Read the model definition and answer for the solid it produces. Units are mm, in the model's axes. A direction names the side the tool comes from. Coordinates: 2 decimals unless noted, no trailing zeros. Loops run counter-clockwise (first coordinate to the right, second up) from the corner with the lowest first, then second, coordinate; pieces in that order, holes last. Notation, with made-up numbers: (-5, 35) - (35, 35) arc R27 cw to (35, 62) - close; hole circle Ø8 at (-24, 55). An arc over 180 degrees is marked (long way). One line per item, written item: value. Start each with the question number.
from build123d import *

# Parameters (mm, degrees)
F0_R     = 10.9855
F1_DEPTH = 6.35


with BuildPart() as f1:
    # F0 (on Front) → F1 (new body)
    with BuildSketch(Plane.XZ):
        with BuildLine():
            ThreePointArc((-22.3335889539, 39.0903010637), (-26.0533328328, 30.1100449426), (-35.0335889539, 26.3903010637))
            ThreePointArc((-35.0335889539, 26.3903010637), (-44.2325232787, 33.2453479745), (-47.7335889539, 44.1703010637))
            ThreePointArc((-47.7335889539, 44.1703010637), (-64.9325473034, 6.0703010637), (-47.7335889539, -32.0296989363))
            ThreePointArc((-47.7335889539, -32.0296989363), (-40.1610226456, -14.7715689431), (-22.3335889539, -8.6585157515))
            ThreePointArc((-22.3335889539, -8.6585157515), (-13.2040635929, -14.2930076328), (-9.6335889539, -24.4096989363))
            ThreePointArc((-9.6335889539, -24.4096989363), (-6.0631143149, -14.2930076328), (3.0664110461, -8.6585157515))
            ThreePointArc((3.0664110461, -8.6585157515), (20.8938447379, -14.7715689431), (28.4664110461, -32.0296989363))
            ThreePointArc((28.4664110461, -32.0296989363), (45.6653693956, 6.0703010637), (28.4664110461, 44.1703010637))
            ThreePointArc((28.4664110461, 44.1703010637), (24.9653453709, 33.2453479745), (15.7664110461, 26.3903010637))
            ThreePointArc((15.7664110461, 26.3903010637), (6.7861549251, 30.1100449426), (3.0664110461, 39.0903010637))
            ThreePointArc((3.0664110461, 39.0903010637), (-0.6533328328, 30.1100449426), (-9.6335889539, 26.3903010637))
            ThreePointArc((-9.6335889539, 26.3903010637), (-18.6138450749, 30.1100449426), (-22.3335889539, 39.0903010637))
        make_face()
        with Locations((-42.6535889539, 8.3668298817)):
            Circle(F0_R, mode=Mode.SUBTRACT)
        with BuildLine():
            ThreePointArc((-9.6335889539, -2.6186701183), (-17.4015104986, 16.1347514264), (1.3519110461, 8.3668298817))
            ThreePointArc((1.3519110461, 8.3668298817), (-1.8656674092, 0.598908337), (-9.6335889539, -2.6186701183))
        make_face(mode=Mode.SUBTRACT)
        with Locations((23.3864110461, 8.3668298817)):
            Circle(F0_R, mode=Mode.SUBTRACT)
    extrude(amount=F1_DEPTH)


solid = f1.part
1) Section A-A, the plane y = -3.75 is taken. Determine the outline of the cut face in (x, z), and give its area (3 significant figures).
2) Section D-D, the plane z = 0 is taken. Determine the outline of the cut face in (x, y), and give its area (3 significant figures).
3) Section C-C, the plane z = -26 is taken. Determine the outline of the cut face in (x, y).
4) Determine the mould class of faces 4 (the cylindrical face through (6.9, -3.1, 30)), 5 (the cylindrical face through (45.66, -3.13, 5.47)), 6 (the cylindrical face through (-44.137, -3.131, 33.113)), 7 (the flat face through (-23, -6.35, 7)) for opening direction X: released by +X, released by -X, zero draft, split by the parting line, or undercut.
5) Flat-ended cylindrical pins translate along their axes: P1, Ø1.5, axis at y = -3, z = -15.5, coming from the -X side; P2, Ø3, axis at x = -15, y = -3, coming from the -Z side; P3, Ø20, axis at x = 23.39, z = 8.37, coming from the -Y side; P4, Ø1.5, axis at x = 13, y = -3, coming from the +Z side. Find the tip coordinate at first contact, or state that the pin passes through.
6) For faces 1 (the cylindrical face through (-40.36, -3.131, -14.957)), 2 (the cylindrical face through (14.67, -3.13, 1.68)), 3 (the cylindrical face through (25.06, -3.13, 33.38)), determine the directions among +Z, -Z, +X, -X, +Y, -Y from which every point of the face is accessible in a straight line to the end or side of a thin tool.
7) Straight lines are drawn through the part: L1, parallel to X at y = -5.25, z = 13; L2, parallel to X at y = -3.5, z = 0; L3, parallel to X at y = -1, z = -19. For each, find the intervals that lie inside material, in ascending order.
8) Section B-B, the plane x = -52 is taken. Determine the outline of the cut face in (y, z), and give its area (3 significant figures).
Answer below:
1. outline: (-47.73, -32.03) arc R23.45 cw to (-22.33, -8.66) arc R16.12 cw to (-9.63, -24.41) arc R16.12 cw to (3.07, -8.66) arc R23.45 cw to (28.47, -32.03) arc R50.8 ccw to (28.47, 44.17) arc R18.8 cw to (15.77, 26.39) arc R12.7 cw to (3.07, 39.09) arc R12.7 cw to (-22.33, 39.09) arc R12.7 cw to (-35.03, 26.39) arc R18.8 cw to (-47.73, 44.17) arc R50.8 ccw to start; hole circle Ø21.97 at (-42.65, 8.37); hole circle Ø21.97 at (-9.63, 8.37); hole circle Ø21.97 at (23.39, 8.37)
1. area: 3,940 mm2
2. outline: (-64.57, -6.35) - (-49.77, -6.35) - (-49.77, 0) - (-64.57, 0) - close; (-35.53, -6.35) - (-16.75, -6.35) - (-16.75, 0) - (-35.53, 0) - close; (-2.51, -6.35) - (16.27, -6.35) - (16.27, 0) - (-2.51, 0) - close; (30.51, -6.35) - (45.3, -6.35) - (45.3, 0) - (30.51, 0) - close
2. area: 426 mm2
3. outline: (-53.53, -6.35) - (-46.95, -6.35) - (-46.95, 0) - (-53.53, 0) - close; (27.68, -6.35) - (34.26, -6.35) - (34.26, 0) - (27.68, 0) - close
4. face 4: undercut
4. face 5: released by +X
4. face 6: undercut
4. face 7: zero draft
5. P1: x = -60.47
5. P2: z = -13.94
5. P3: through
5. P4: z = 26.89
6. face 1: -Z, +Y, -Y
6. face 2: +Y, -Y
6. face 3: +Z, +Y, -Y
7. L1: -64.46 to -52.61, -32.69 to -19.59, 0.33 to 13.43, 33.35 to 45.19
7. L2: -64.57 to -49.77, -35.53 to -16.75, -2.51 to 16.27, 30.51 to 45.3
7. L3: -58.32 to -43.78, -10.57 to -8.7, 24.51 to 39.05
8. outline: (-6.35, -27.79) - (0, -27.79) - (0, 2.59) - (-6.35, 2.59) - close; (-6.35, 14.14) - (0, 14.14) - (0, 39.93) - (-6.35, 39.93) - close
8. area: 357 mm2
